```python
from build123d import *

# Parameters (mm, degrees)
BOSS_EXTRUDE1_DEPTH         = 289.71875
CUT_TOP_RIGHT_FRONT_DEPTH   = 27.162
CUT_FRONT_LEFT_BOTTOM_DEPTH = 16.24


with BuildPart() as part:
    # Sketch1 → Boss-Extrude1 (new body, symmetric)
    with BuildSketch(Plane(origin=(0, 0, 0), x_dir=(0, 0, -1), z_dir=(1, 0, 0))):
        with BuildLine():
            Line((7.62, 0), (7.62, -21.844))
            Line((7.62, -21.844), (2.54, -21.844))
            Line((2.54, -21.844), (2.202186415, -24.247668555))
            ThreePointArc((2.202186415, -24.247668555), (0, -26.162), (-2.202186415, -24.247668555))
            Line((-2.202186415, -24.247668555), (-2.54, -21.844))
            Line((-2.54, -21.844), (-7.62, -21.844))
            Line((-7.62, -21.844), (-7.62, -7.874))
            Line((-7.62, -7.874), (-6.35, -7.874))
            Line((-6.35, -7.874), (-6.35, -20.574))
            Line((-6.35, -20.574), (-1.436005843, -20.574))
            Line((-1.436005843, -20.574), (-0.944545968, -24.070918717))
            ThreePointArc((-0.944545968, -24.070918717), (0, -24.892), (0.944545968, -24.070918717))
            Line((0.944545968, -24.070918717), (1.436005843, -20.574))
            Line((1.436005843, -20.574), (6.35, -20.574))
            Line((6.35, -20.574), (6.35, 0))
            Line((6.35, 0), (7.62, 0))
        make_face()
    extrude(amount=BOSS_EXTRUDE1_DEPTH, both=True)

    # Sketch2 → Cut-Top-Right-Front (cut, through all)
    with BuildSketch(Plane(origin=(0, 0, 0), x_dir=(1, 0, 0), z_dir=(0, 1, 0))):
        Polygon((289.71875, 7.62), (274.47875, -7.62), (289.71875, -7.62), align=None)
    extrude(amount=-CUT_TOP_RIGHT_FRONT_DEPTH, mode=Mode.SUBTRACT)

    # Sketch12 → Cut-Front-Left-Bottom (cut, through all)
    with BuildSketch(Plane.XY.offset(7.62)):
        Polygon((-289.71875, 0), (-263.55675, -26.162), (-289.71875, -26.162), align=None)
    extrude(amount=-CUT_FRONT_LEFT_BOTTOM_DEPTH, mode=Mode.SUBTRACT)


solid = part.part
```
Source: CAD feature listing. Evaluate the final solid. Frame: model axes, mm. A direction names the side the tool comes from. Coordinates: 2 decimals unless noted, no trailing zeros. Write each loop counter-clockwise with the first axis right and the second up, starting at its lowest first coordinate (ties: lowest second). Pieces come first, ordered by that corner, then holes. Notation, with made-up numbers: (2, 54.5) - (8, 54.5) arc R27 cw to (8, 72.5) - close; hole circle Ø11 at (72.5, -0.75). An arc over 180 degrees is marked (long way). Answer as a JSON object with one key per item and string values.
Q1. Section query B-B, the plane x = 185.5. Output: boundary loops of the cut face in (y, z).
Ans:
{"outline": "(-24.25, -2.2) - (-21.84, -2.54) - (-21.84, -7.62) - (0, -7.62) - (0, -6.35) - (-20.57, -6.35) - (-20.57, -1.44) - (-24.07, -0.94) arc R0.95 cw to (-24.07, 0.94) - (-20.57, 1.44) - (-20.57, 6.35) - (-7.87, 6.35) - (-7.87, 7.62) - (-21.84, 7.62) - (-21.84, 2.54) - (-24.25, 2.2) arc R2.22 ccw to start"}
Q2. Set-up query: faces 1 (the flat face through (-273.79, -15.93, -6.74)), 2 (the flat face through (3, -10, -6.35)). Return all of +Z, -Z, +X, -X, +Y, -Y with unobstructed straight access to the full face (end or side cutting, diameter ignored); none if empty.
Ans:
{"face 1": "+Z, -Z, -X, -Y", "face 2": "+X, -X, +Y"}
Q3. Material intervals for line 1 (Z direction, x = -189.5, y = -10.75); line 2 (Y direction, x = 165.5, z = 6); line 3 (Z direction, x = -110.5, y = -22.75), sorted ascending. Write a range as [from, to].
Ans:
{"line 1": "z = [-7.62, -6.35], [6.35, 7.62]", "line 2": "y = [-21.84, -20.57]", "line 3": "z = [-2.41, -1.13], [1.13, 2.41]"}
Q4. Section query A-A, the plane y = -14.5. Output: boundary loops of the cut face in (x, z), plus the area to 3 significant figures.
Ans:
{"outline": "(-275.22, -7.62) - (289.72, -7.62) - (288.45, -6.35) - (-275.22, -6.35) - close; (-275.22, 6.35) - (275.75, 6.35) - (274.48, 7.62) - (-275.22, 7.62) - close", "area": "1,420 mm2"}
Q5. First-contact query: pin 1 Ø4 at (x, z) = (-122.5, -5.5) entering from -Y; pin 2 Ø4 at (x, z) = (-98, -3) entering from +Y; pin 3 Ø8 at (x, z) = (147.5, 4.5) entering from +Y. Flat tips, straight axial feed; report the tip coordinate or a pass-through.
Ans:
{"pin 1": "stops at y = -21.84", "pin 2": "stops at y = -20.57", "pin 3": "stops at y = -7.87"}
